```python
from build123d import *

# Parameters (mm, degrees)
SKETCH1_W                      = 96
SKETCH1_H                      = 121.5
SKETCH1_W_2                    = 86
SKETCH1_H_2                    = 98.5
BOSS_EXTRUDE1_DEPTH            = 2
SKETCH2_W                      = 100
SKETCH2_H                      = 125.5
SKETCH2_W_2                    = 96
SKETCH2_H_2                    = 121.5
BOSS_EXTRUDE2_DEPTH            = 2
SKETCH8_W                      = 100
SKETCH8_H                      = 2
BOSS_EXTRUDE6_DEPTH            = 10
CUT_EXTRUDE1_REACH             = 14
SKETCH3_R                      = 2.25
SKETCH3_R_2                    = 1.65
CUT_EXTRUDE1_DIRECTION_2_DEPTH = 1


with BuildPart() as part:
    # Sketch1 → Boss-Extrude1 (new body)
    with BuildSketch(Plane(origin=(0, 0, 0), x_dir=(1, 0, 0), z_dir=(0, 1, 0))):
        Rectangle(SKETCH1_W, SKETCH1_H)
        with Locations((0, 6.5)):
            Rectangle(SKETCH1_W_2, SKETCH1_H_2, mode=Mode.SUBTRACT)
    extrude(amount=BOSS_EXTRUDE1_DEPTH)

    # Sketch2 → Boss-Extrude2 (add)
    with BuildSketch(Plane(origin=(0, 0, 0), x_dir=(1, 0, 0), z_dir=(0, 1, 0))):
        Rectangle(SKETCH2_W, SKETCH2_H)
        Rectangle(SKETCH2_W_2, SKETCH2_H_2, mode=Mode.SUBTRACT)
    extrude(amount=BOSS_EXTRUDE2_DEPTH)

    # Sketch8 → Boss-Extrude6 (add)
    with BuildSketch(Plane(origin=(0, 2, 0), x_dir=(1, 0, 0), z_dir=(0, 1, 0))):
        with Locations((0, 61.75)):
            Rectangle(SKETCH8_W, SKETCH8_H)
    extrude(amount=BOSS_EXTRUDE6_DEPTH)

    # Sketch3 → Cut-Extrude1 (cut, up to next)
    with BuildSketch(Plane.XZ, mode=Mode.PRIVATE) as cut_extrude1_sk1:
        with Locations((25, 52.75)):
            Circle(SKETCH3_R)
    cut_extrude1_tool1 = extrude(cut_extrude1_sk1.sketch, amount=-CUT_EXTRUDE1_REACH, mode=Mode.PRIVATE) & part.part
    add(cut_extrude1_tool1.solids().sort_by_distance((25, 0, 52.75))[0], mode=Mode.SUBTRACT)
    # Sketch3 → Cut-Extrude1 (cut, up to next)
    with BuildSketch(Plane.XZ, mode=Mode.PRIVATE) as cut_extrude1_sk2:
        with Locations((-25, 52.75)):
            Circle(SKETCH3_R)
    cut_extrude1_tool2 = extrude(cut_extrude1_sk2.sketch, amount=-CUT_EXTRUDE1_REACH, mode=Mode.PRIVATE) & part.part
    add(cut_extrude1_tool2.solids().sort_by_distance((-25, 0, 52.75))[0], mode=Mode.SUBTRACT)
    # Sketch3 → Cut-Extrude1 (cut, up to next)
    with BuildSketch(Plane.XZ, mode=Mode.PRIVATE) as cut_extrude1_sk3:
        with Locations((46.5, -59.25)):
            Circle(SKETCH3_R_2)
    cut_extrude1_tool3 = extrude(cut_extrude1_sk3.sketch, amount=-CUT_EXTRUDE1_REACH, mode=Mode.PRIVATE) & part.part
    add(cut_extrude1_tool3.solids().sort_by_distance((46.5, 0, -59.25))[0], mode=Mode.SUBTRACT)
    # Sketch3 → Cut-Extrude1 (cut, up to next)
    with BuildSketch(Plane.XZ, mode=Mode.PRIVATE) as cut_extrude1_sk4:
        with Locations((-46.5, -59.25)):
            Circle(SKETCH3_R_2)
    cut_extrude1_tool4 = extrude(cut_extrude1_sk4.sketch, amount=-CUT_EXTRUDE1_REACH, mode=Mode.PRIVATE) & part.part
    add(cut_extrude1_tool4.solids().sort_by_distance((-46.5, 0, -59.25))[0], mode=Mode.SUBTRACT)

    # Sketch3 → Cut-Extrude1 direction 2 (cut)
    with BuildSketch(Plane.XZ):
        with Locations((25, 52.75)):
            Circle(SKETCH3_R)
        with Locations((-25, 52.75)):
            Circle(SKETCH3_R)
        with Locations((46.5, -59.25)):
            Circle(SKETCH3_R_2)
        with Locations((-46.5, -59.25)):
            Circle(SKETCH3_R_2)
    extrude(amount=CUT_EXTRUDE1_DIRECTION_2_DEPTH, mode=Mode.SUBTRACT)


solid = part.part
```
The listing builds one solid part. Answer for the finished solid, in the listing's coordinates (mm). A direction names the side the tool comes from. Give positions to 0.01 mm unless a question says otherwise; leave off trailing zeros. Order: outer loops, then holes, each group sorted by start corner. A loop starts at its lowest first (then second) coordinate and runs counter-clockwise, first axis right, second up. Notation, with made-up numbers: (20, -27) -> (50, -27) arc R26 cw to (50, -3) -> close; hole circle Ø10 at (74.25, -13). An arc over 180 degrees is marked (long way). Answer as CSV lines item,"result". Start each with the question number.
Q1. Determine the mould class of faces 3 (the flat face through (49, 7, -60.75)), 4 (the flat face through (50, 1, 0)), 5 (the cylindrical face through (-46.43, 2.86, -60.9)) for opening direction X: pulls with the +X half, pulls with the -X half, needs draft (parallel to the pull), parting line crosses it, or undercut.
Q2. Which of the six approach directions +Z, -Z, +X, -X, +Y, -Y give full straight-line access (tool end or side, diameter ignored) to faces 1 (the cylindrical face through (26.21, 0.986, 54.647)), 2 (the flat face through (-15, 2, 46))?
Q3. A cutting plane is placed at A-A (z = 5). Determine the outline of the cut face in (x, y), then the cut area to 3 significant figures.
Q4. Find the intervals of material crossed by L1, parallel to Z at x = 25, y = 0.85; L2, parallel to Z at x = -18, y = 5.25; L3, parallel to Z at x = 46.5, y = 7.5, in increasing order.
Q5. A cutting plane is placed at D-D (y = 5.25). Determine the outline of the cut face in (x, z), then the cut area to 3 significant figures.
Q6. A cutting plane is placed at C-C (z = -59.25). Determine the outline of the cut face in (x, y).
Q7. A cutting plane is placed at B-B (x = 25). Determine the outline of the cut face in (y, z).
Q8. Given pin 1 (2.5 mm diameter, centred on x = 49, y = 7.5, fed in from +Z); pin 2 (4.5 mm diameter, centred on x = 46.5, z = -59.25, fed in from +Y); pin 3 (6 mm diameter, centred on x = -25, z = 52.75, fed in from +Y), each flat-ended and moving along its own axis, determine where each tip first touches the part or whether it passes through.
Results found:
1,face 3,"needs draft"
1,face 4,"pulls with the +X half"
1,face 5,"undercut"
2,face 1,"+Y, -Y"
2,face 2,"+Z, +X, -X, +Y"
3,outline,"(-50, 0) -> (-43, 0) -> (-43, 2) -> (-50, 2) -> close; (43, 0) -> (50, 0) -> (50, 2) -> (43, 2) -> close"
3,area,"28.0 mm2"
4,L1,"-62.75 to -55.75, 42.75 to 50.5, 55 to 62.75"
4,L2,"-62.75 to -60.75"
4,L3,"-62.75 to -60.9"
5,outline,"(-50, -62.75) -> (50, -62.75) -> (50, -60.75) -> (47.19, -60.75) arc R1.65 cw to (45.81, -60.75) -> (-45.81, -60.75) arc R1.65 cw to (-47.19, -60.75) -> (-50, -60.75) -> close"
5,area,"200 mm2"
6,outline,"(-50, 0) -> (-48.15, 0) -> (-48.15, 2) -> (-50, 2) -> close; (-44.85, 0) -> (44.85, 0) -> (44.85, 2) -> (-44.85, 2) -> close; (48.15, 0) -> (50, 0) -> (50, 2) -> (48.15, 2) -> close"
7,outline,"(0, -62.75) -> (12, -62.75) -> (12, -60.75) -> (2, -60.75) -> (2, -55.75) -> (0, -55.75) -> close; (0, 42.75) -> (2, 42.75) -> (2, 50.5) -> (0, 50.5) -> close; (0, 55) -> (2, 55) -> (2, 62.75) -> (0, 62.75) -> close"
8,pin 1,"z = -60.75"
8,pin 2,"y = 12"
8,pin 3,"y = 2"
